Can you work these out from the model? Positions are in its coordinate system, mm. A direction names the side the tool comes from. Coordinates: 2 decimals unless noted, no trailing zeros. Loops run counter-clockwise (first coordinate to the right, second up) from the corner with the lowest first, then second, coordinate; pieces in that order, holes last. Notation, with made-up numbers: (81.25, -36) -> (125.25, -36) arc R26 ccw to (125.25, -13) -> close; hole circle Ø11 at (-35.75, -8). An arc over 180 degrees is marked (long way). Use one line per item in the form item = value. Start each with the question number.
(1) I need wall thicknesses on line 1 (Y direction, x = -125, z = -70); line 2 (Y direction, x = 127, z = -69.25); line 3 (X direction, y = 33.5, z = -69.25). Which ranges of each line are inside material? Lowest first, please. Write a range as [from, to].
(2) Imagine slicing it at B-B (x = 0). List the corners of the cut face in (y, z) for me.
(3) Imagine slicing it at A-A (z = -68). State how many separate pieces and enclosed holes the cut face has, plus the area to 3 significant figures.
(4) Imagine slicing it at D-D (x = 73). List the corners of the cut face in (y, z) for me, plus the area to 3 significant figures.
(5) Imagine slicing it at C-C (y = 44). List the corners of the cut face in (x, z) for me.
(6) Thinking about a two-plate mould opening in X: for faces 1 (the flat face through (-98.28, 85.26, -68.7)), 2 (the cylindrical face through (-105.01, 35.13, -68.7)), 3 (the cylindrical face through (0.99, 149.99, -68.7)), which applies, released by +X, released by -X, zero draft, split by the parting line, or undercut?
(7) I'm going to push flat-ended pins straight in: pin 1 (13.5 mm diameter, centred on x = -127, y = 19, fed in from -Z); pin 2 (3 mm diameter, centred on y = 111.5, z = -71.5, fed in from +X); pin 3 (5 mm diameter, centred on x = -87.5, z = -65.5, fed in from +Y); pin 4 (2 mm diameter, centred on y = 102.5, z = -70, fed in from +X). Where does each tip first touch, or does it pass through?
(8) On a 3-axis mill with a long thin cutter (end or side, diameter ignored), from which of +Z, -Z, +X, -X, +Y, -Y can I reach the whole of each face in a straight line? I mean faces 4 (the cylindrical face through (122.24, 17.03, -68.83)), 5 (the flat face through (-108, 23, -69)). Say none if no direction works.
```python
from build123d import *

# Parameters (mm, degrees)
F1_DEPTH = 9.525
F2_D     = 10.3
F3_D     = 8.8
F4_D     = 12
F5_ANGLE = 90


# Not quite as in the source:
# - a length typed as a fraction of an inch, garbled in the dataset ("3 / 203.2 mm" for 3/8 in), is restored
# - a feature names something its author has since deleted; it is built from what else it names


with BuildPart() as f1:
    # F0 (on Front) → F1 (new body)
    with BuildSketch(Plane.XZ):
        with BuildLine():
            ThreePointArc((-108, -36.0045329175), (-104.9318381582, -28.796924455), (-97.6100760503, -26.0121378435))
            Line((-97.6100760503, -26.0121378435), (0, -26.0121378435))
            Line((0, -26.0121378435), (97.6100760503, -26.0121378435))
            ThreePointArc((97.6100760503, -26.0121378435), (104.9318381582, -28.796924455), (108, -36.0045329175))
            Line((108, -36.0045329175), (108, -45.0045329175))
            ThreePointArc((108, -45.0045329175), (127.1790782013, -64.0036889776), (145.9966243156, -44.6463924235))
            Line((145.9966243156, -44.6463924235), (145, 10.9954670825))
            Line((145, 10.9954670825), (52.8553396226, 31.2281526171))
            ThreePointArc((52.8553396226, 31.2281526171), (47.2074842389, 34.7283546603), (45, 40.9954670825))
            ThreePointArc((45, 40.9954670825), (31.8198051534, 72.8152722359), (0, 85.9954670825))
            ThreePointArc((0, 85.9954670825), (-31.8198051534, 72.8152722359), (-45, 40.9954670825))
            ThreePointArc((-45, 40.9954670825), (-47.2074842389, 34.7283546603), (-52.8553396226, 31.2281526171))
            Line((-52.8553396226, 31.2281526171), (-145, 10.9954670825))
            Line((-145, 10.9954670825), (-145.9966243156, -44.6463924235))
            ThreePointArc((-145.9966243156, -44.6463924235), (-127.1790782013, -64.0036889776), (-108, -45.0045329175))
            Line((-108, -45.0045329175), (-108, -36.0045329175))
        make_face()
    extrude(amount=-F1_DEPTH)

    # F2 (through all)
    with Locations(Plane.XZ):
        with Locations((-127, -45.0045329175), (-127, -20.0045329175), (127, -45.0045329175)):
            Hole(F2_D / 2)

    # F3 (through all)
    with Locations(Plane.XZ):
        with Locations((-60, -7.0045329175), (-35, -7.0045329175), (35, -7.0045329175), (60, -7.0045329175)):
            Hole(F3_D / 2)

    # F4 (through all)
    with Locations(Plane.XZ):
        with Locations((0, 40.9954670825)):
            Hole(F4_D / 2)


with BuildPart() as f1_1:
    # F5: moved
    add(f1.part.rotate(Axis((-53.975, 0, -64.0045329175), (-1, 0, 0)), F5_ANGLE))


solid = f1_1.part
```
Worked out:
q1.line_1 = [0.11, 14.25], [23.75, 39.25], [48.75, 79.39]
q1.line_2 = [0, 13.85], [24.15, 78.95]
q1.line_3 = [-145.74, -106.35], [106.35, 145.74]
q2.outline = (37.99, -73.53) -> (99, -73.53) -> (99, -64) -> (37.99, -64) -> close; (111, -73.53) -> (150, -73.53) -> (150, -64) -> (111, -64) -> close
q3.separate_pieces = 1
q3.enclosed_holes = 8
q3.area = 20,900 mm2
q4.outline = (37.99, -73.53) -> (90.81, -73.53) -> (90.81, -64) -> (37.99, -64) -> close
q4.area = 503 mm2
q5.outline = (-145.56, -73.53) -> (-132.15, -73.53) -> (-132.15, -64) -> (-145.56, -64) -> close; (-121.85, -73.53) -> (145.56, -73.53) -> (145.56, -64) -> (-121.85, -64) -> close
q6.face_1 = released by -X
q6.face_2 = undercut
q6.face_3 = split by the parting line
q7.pin_1 = -73.53
q7.pin_2 = 44.72
q7.pin_3 = 88.17
q7.pin_4 = 45.63
q8.face_4 = +Z, -Z
q8.face_5 = +Z, -Z, -Y
